```python
from build123d import *

# Parameters (mm, degrees)
F0_W      = 180
F0_H      = 90
F1_DEPTH  = 75
F2_W      = 80
F2_H      = 68
F3_DEPTH  = 175
F4_W      = 80
F4_H      = 68
F5_DEPTH  = 5
F7_DEPTH  = 25
F9_DEPTH  = 1
F10_DEPTH = 0.5


with BuildPart() as f1:
    # F0 (on Top) → F1 (new body)
    with BuildSketch(Plane.XY):
        Rectangle(F0_W, F0_H)
    extrude(amount=F1_DEPTH)

    # F2 (on face) → F3 (cut)
    with BuildSketch(Plane(origin=(-90, 0, 0), x_dir=(0, -1, 0), z_dir=(-1, 0, 0))):
        with Locations((0, 39)):
            Rectangle(F2_W, F2_H)
    extrude(amount=-F3_DEPTH, mode=Mode.SUBTRACT)

    # F4 (on face) → F5 (join)
    with BuildSketch(Plane(origin=(-90, 0, 0), x_dir=(0, -1, 0), z_dir=(-1, 0, 0))):
        with Locations((0, 39)):
            Rectangle(F4_W, F4_H)
    extrude(amount=-F5_DEPTH)

    # F6 (on face) → F7 (cut, symmetric)
    with BuildSketch(Plane.XY.offset(75)):
        with BuildLine():
            ThreePointArc((53.4038208425, -7.8985784203), (1.5108137294, 15.9196343033), (-53.3230871735, 0))
            ThreePointArc((-53.3230871735, 0), (-1.0370293111, -18.5072454911), (53.4038208425, -7.8985784203))
        make_face()
    extrude(amount=F7_DEPTH, both=True, mode=Mode.SUBTRACT)

    # F8 (on face) → F9 (cut)
    with BuildSketch(Plane.XZ.offset(45)):
        Polygon((-81.387918066, 14.9286104324), (-81.387918066, 5), (-78.8312283214, 5), (-78.8312283214, 14.9286104324), (-75.5595097627, 14.9286104324), (-75.5595097627, 17.0552274955), (-84.6622751074, 17.0552274955), (-84.6622751074, 14.9286104324), align=None)
        with BuildLine():
            add(Edge.make_bspline(
                [(-71.3481548896, 5), (-71.8881241204, 5.1447529863), (-72.3603494786, 5.4155610266)],
                knots=[0.5345224838, 0.5345224838, 0.5345224838, 1, 1, 1], degree=2))
            Line((-71.3481548896, 5), (-68.6078073449, 5))
            add(Edge.make_bspline(
                [(-66.7126772409, 6.1042050135), (-67.4705184641, 5.2933149046), (-68.6078073449, 5)],
                knots=[0, 0, 0, 0.6382803275, 0.6382803275, 0.6382803275], degree=2))
            add(Edge.make_bspline(
                [(-65.525360022, 9.6252601882), (-65.525360022, 7.3746344377), (-66.7126772409, 6.1042050135)],
                knots=[0, 0, 0, 1, 1, 1], degree=2))
            add(Edge.make_bspline(
                [(-66.06888746, 12.156884347), (-65.525360022, 11.0764256779), (-65.525360022, 9.6252601882)],
                knots=[0, 0, 0, 1, 1, 1], degree=2))
            add(Edge.make_bspline(
                [(-67.6269114994, 13.813851488), (-66.6124148979, 13.2373430162), (-66.06888746, 12.156884347)],
                knots=[0, 0, 0, 1, 1, 1], degree=2))
            add(Edge.make_bspline(
                [(-69.9685649032, 14.3903599599), (-68.6414081008, 14.3903599599), (-67.6269114994, 13.813851488)],
                knots=[0, 0, 0, 1, 1, 1], degree=2))
            add(Edge.make_bspline(
                [(-73.2838184266, 13.1370806733), (-72.1057358972, 14.3903599599), (-69.9685649032, 14.3903599599)],
                knots=[0, 0, 0, 1, 1, 1], degree=2))
            add(Edge.make_bspline(
                [(-74.461900956, 9.6252601882), (-74.461900956, 11.8838013867), (-73.2838184266, 13.1370806733)],
                knots=[0, 0, 0, 1, 1, 1], degree=2))
            add(Edge.make_bspline(
                [(-73.918373518, 7.0857205811), (-74.461900956, 8.1740946984), (-74.461900956, 9.6252601882)],
                knots=[0, 0, 0, 1, 1, 1], degree=2))
            add(Edge.make_bspline(
                [(-72.3603494786, 5.4155610266), (-73.37484608, 5.9973464638), (-73.918373518, 7.0857205811)],
                knots=[0, 0, 0, 1, 1, 1], degree=2))
        make_face()
        with BuildLine():
            add(Edge.make_bspline(
                [(-71.8999342459, 9.6252601882), (-71.8999342459, 8.2558876624), (-71.4500729441, 7.5553705033)],
                knots=[0, 0, 0, 1, 1, 1], degree=2))
            add(Edge.make_bspline(
                [(-71.4540306682, 11.6832767009), (-71.8999342459, 11.002548162), (-71.8999342459, 9.6252601882)],
                knots=[0, 0, 0, 1, 1, 1], degree=2))
            add(Edge.make_bspline(
                [(-70.0028651785, 12.3640052397), (-71.0081270904, 12.3640052397), (-71.4540306682, 11.6832767009)],
                knots=[0, 0, 0, 1, 1, 1], degree=2))
            add(Edge.make_bspline(
                [(-68.5424649993, 11.6793189768), (-68.9870493357, 12.3640052397), (-70.0028651785, 12.3640052397)],
                knots=[0, 0, 0, 1, 1, 1], degree=2))
            add(Edge.make_bspline(
                [(-68.0978806629, 9.6252601882), (-68.0978806629, 10.9946327139), (-68.5424649993, 11.6793189768)],
                knots=[0, 0, 0, 1, 1, 1], degree=2))
            add(Edge.make_bspline(
                [(-68.5385072752, 7.5514127792), (-68.0978806629, 8.2479722143), (-68.0978806629, 9.6252601882)],
                knots=[0, 0, 0, 1, 1, 1], degree=2))
            add(Edge.make_bspline(
                [(-69.9870342822, 6.8548533441), (-68.9791338875, 6.8548533441), (-68.5385072752, 7.5514127792)],
                knots=[0, 0, 0, 1, 1, 1], degree=2))
            add(Edge.make_bspline(
                [(-71.4500729441, 7.5553705033), (-71.0002116423, 6.8548533441), (-69.9870342822, 6.8548533441)],
                knots=[0, 0, 0, 1, 1, 1], degree=2))
        make_face(mode=Mode.SUBTRACT)
        with BuildLine():
            Line((-63.4462356476, 5), (-60.9317616263, 5))
            Line((-60.9317616263, 5), (-60.9317616263, 9.6912222559))
            add(Edge.make_bspline(
                [(-60.2589485356, 11.4233861541), (-60.9317616263, 10.8046619589), (-60.9317616263, 9.6912222559)],
                knots=[0, 0, 0, 1, 1, 1], degree=2))
            add(Edge.make_bspline(
                [(-58.3829873298, 12.0421103492), (-59.586135445, 12.0421103492), (-60.2589485356, 11.4233861541)],
                knots=[0, 0, 0, 1, 1, 1], degree=2))
            add(Edge.make_bspline(
                [(-57.6415736887, 11.9603173853), (-57.9476376829, 12.0421103492), (-58.3829873298, 12.0421103492)],
                knots=[0, 0, 0, 1, 1, 1], degree=2))
            Line((-57.6415736887, 11.9603173853), (-57.4516029337, 14.316482444))
            add(Edge.make_bspline(
                [(-58.3011943659, 14.3903599599), (-57.7893287204, 14.3903599599), (-57.4516029337, 14.316482444)],
                knots=[0, 0, 0, 1, 1, 1], degree=2))
            add(Edge.make_bspline(
                [(-59.8882417151, 13.9167523137), (-59.1587012462, 14.3903599599), (-58.3011943659, 14.3903599599)],
                knots=[0, 0, 0, 1, 1, 1], degree=2))
            add(Edge.make_bspline(
                [(-61.0478548655, 12.6674307512), (-60.617782184, 13.4431446675), (-59.8882417151, 13.9167523137)],
                knots=[0, 0, 0, 1, 1, 1], degree=2))
            Line((-61.0478548655, 12.6674307512), (-61.1692250701, 12.6674307512))
            Line((-61.1692250701, 12.6674307512), (-61.541251132, 14.2188585838))
            Line((-61.541251132, 14.2188585838), (-63.4462356476, 14.2188585838))
            Line((-63.4462356476, 14.2188585838), (-63.4462356476, 5))
        make_face()
        Polygon((-49.5282393598, 5), (-46.6259083804, 5), (-50.5097549274, 10.2189187976), (-46.8501794106, 14.2188585838), (-49.6865483223, 14.2188585838), (-52.2669844113, 11.4141514646), (-53.3619547354, 10.0131171463), (-53.3962550106, 10.0131171463), (-53.2643308752, 12.1080724169), (-53.2643308752, 17.8309414119), (-55.7788048965, 17.8309414119), (-55.7788048965, 5), (-53.2643308752, 5), (-53.2643308752, 7.8706691869), (-52.1825529647, 8.7360915154), align=None)
    extrude(amount=-F9_DEPTH, mode=Mode.SUBTRACT)

    # F10 (cut): a face of the model
    f10_faces = [f1.faces().sort_by_distance(p)[0] for p in [
        (-69.997731823, -45, 9.6131266582),
    ]]
    extrude(f10_faces, amount=-F10_DEPTH, mode=Mode.SUBTRACT)


solid = f1.part
```
Could you check a few things on this model? Use its own coordinates, in mm. A direction names the side the tool comes from. Round coordinates to 2 decimals unless told otherwise and drop trailing zeros. Loops run counter-clockwise (first coordinate to the right, second up) from the corner with the lowest first, then second, coordinate; pieces in that order, holes last. Notation, with made-up numbers: (68.25, 9) - (74.25, 9) arc R7 ccw to (74.25, 18) - close; hole circle Ø7 at (-0.5, -24). An arc over 180 degrees is marked (long way). Answer in a Markdown table with one row per item. Add a question column.
(1) If we section it at C-C (y = -3.5): Please give me the cut outline in (x, z), plus the area to 3 significant figures.
(2) If we mould it in two halves opening along Z, with no side actions, what happens to faces 1 (the face through (-1, 1, 0)), 2 (the face through (-1, 1, 5)), 3 (the face through (-90, 1, 38))? For each: pulls with the +Z half, pulls with the -Z half, needs draft (parallel to the pull), parting line crosses it, or undercut.
(3) For faces 4 (the face through (-67.9, -44, 9.8)), 5 (the face through (-1, 21, 75)), 6 (the face through (-1, -40, 39)), which set-ups out of +Z, -Z, +X, -X, +Y, -Y let a thin tool reach every point of the face, with its end or its side?
(4) If we section it at A-A (x = 60.5): Please give me the cut outline in (y, z).
(5) I need wall thicknesses on line 1 along Y through (x, z) = (-65, 55); line 2 along Z through (x, y) = (-58, -17.5); line 3 along X through (y, z) = (13, 46). Which ranges of each line are inside material? Lowest first, please.
(6) If we section it at B-B (z = 28): Please give me the cut outline in (x, y), plus the area to 3 significant figures.
(7) If we section it at D-D (x = 35.5): Please give me the cut outline in (y, z).
Model answer:
| question | item | result |
|---|---|---|
| 1 | outline | (-90, 0) - (90, 0) - (90, 75) - (48.66, 75) - (48.66, 73) - (85, 73) - (85, 5) - (-85, 5) - (-85, 73) - (-47.93, 73) - (-47.93, 75) - (-90, 75) - close |
| 1 | area | 1,750 mm² |
| 2 | face 1 | pulls with the -Z half |
| 2 | face 2 | undercut |
| 2 | face 3 | needs draft |
| 3 | face 4 | -Y |
| 3 | face 5 | +Z, +X, -X, +Y, -Y |
| 3 | face 6 | none |
| 4 | outline | (-45, 0) - (45, 0) - (45, 75) - (-45, 75) - close; hole (-40, 5) - (40, 5) - (40, 73) - (-40, 73) - close |
| 5 | line 1 | y = -45 to -40, 40 to 45 |
| 5 | line 2 | z = 0 to 5, 73 to 75 |
| 5 | line 3 | x = -90 to -85, 85 to 90 |
| 6 | outline | (-90, -45) - (90, -45) - (90, 45) - (-90, 45) - close; hole (-85, -40) - (85, -40) - (85, 40) - (-85, 40) - close |
| 6 | area | 2,600 mm² |
| 7 | outline | (-45, 0) - (45, 0) - (45, 75) - (5.68, 75) - (5.68, 73) - (40, 73) - (40, 5) - (-40, 5) - (-40, 73) - (-14.79, 73) - (-14.79, 75) - (-45, 75) - close |
